The listing builds one solid part. Answer for the finished solid, in the listing's coordinates (mm). Coordinates: 2 decimals unless noted, no trailing zeros. Order: outer loops, then holes, each group sorted by start corner. A loop starts at its lowest first (then second) coordinate and runs counter-clockwise, first axis right, second up. Notation, with made-up numbers: (20, -9.75) - (58, -9.75) arc R6 cw to (58, 0.25) - close; hole circle Ø10 at (28.5, 12.5). An arc over 180 degrees is marked (long way). Use a Markdown table: item, result. Add a question column.
Item 1: The part is cut by section D-D, the plane y = 165.5. Give the vertices of the cut face in (x, z), then the cut area to 3 significant figures.
Item 2: Find the intervals of material crossed by line 1 along Z through (x, y) = (72, 80); line 2 along Y through (x, z) = (0, -162); line 3 along Y through (x, z) = (0, 104), in increasing order.
Item 3: The part is cut by section C-C, the plane y = 34. Give the vertices of the cut face in (x, z).
Item 4: Flat-ended cylindrical pins translate along their axes: P1, Ø17, axis at x = 197.99, y = 197.99, coming from the +Z side; P2, Ø15, axis at x = 77.78, y = -77.78, coming from the -Z side; P3, Ø21, axis at x = -77.78, y = 77.78, coming from the -Z side. Find the tip coordinate at first contact, or state that the pin passes through.
Item 5: The part is cut by section A-A, the plane x = 134. Give the vertices of the cut face in (y, z), then the cut area to 3 significant figures.
Item 6: The part is cut by section B-B, the plane z = 136. Give the vertices of the cut face in (x, y), then the cut area to 3 significant figures.
from build123d import *

# Parameters (mm, degrees)
SKETCH1_R               = 17.5
SKETCH1_R_2             = 6.5
BOSS_EXTRUDE1_DEPTH     = 280
SKETCH2_R               = 6.5
BOSS_EXTRUDE2_DEPTH     = 10
SKETCH3_R               = 6.5
BOSS_EXTRUDE3_DEPTH     = 10
MIRROR3_COPY_1_SKETCH_R = 6.5
MIRROR3_COPY_1_DEPTH    = 10
SKETCH4_R               = 6.5
BOSS_EXTRUDE4_DEPTH     = 5


with BuildPart() as part:
    # Sketch1 → Boss-Extrude1 (new, symmetric)
    with BuildSketch(Plane.XY):
        Circle(SKETCH1_R)
        Circle(SKETCH1_R_2, mode=Mode.SUBTRACT)
    extrude(amount=BOSS_EXTRUDE1_DEPTH, both=True)

    # Sketch2 → Boss-Extrude2 (add)
    with BuildSketch(Plane.XY.offset(210)):
        with BuildLine():
            Line((-12.374368671, 12.374368671), (192.686597873, 217.435335215))
            ThreePointArc((192.686597873, 217.435335215), (199.757665685, 220.364267403), (206.828733497, 217.435335215))
            Line((206.828733497, 217.435335215), (217.435335215, 206.828733497))
            ThreePointArc((217.435335215, 206.828733497), (220.364267403, 199.757665685), (217.435335215, 192.686597873))
            Line((217.435335215, 192.686597873), (12.374368671, -12.374368671))
            ThreePointArc((12.374368671, -12.374368671), (12.374368671, 12.374368671), (-12.374368671, 12.374368671))
        make_face()
        with Locations((197.989898732, 197.989898732)):
            Circle(SKETCH2_R, mode=Mode.SUBTRACT)
    boss_extrude2 = extrude(amount=-BOSS_EXTRUDE2_DEPTH)

    # Mirror1: Boss-Extrude2 across plane
    add(boss_extrude2.mirror(Plane.XY))

    # Sketch3 → Boss-Extrude3 (add)
    with BuildSketch(Plane.XY.offset(130)):
        with BuildLine():
            Line((12.374368671, 12.374368671), (-72.478445072, 97.227182413))
            ThreePointArc((-72.478445072, 97.227182413), (-79.549512883, 100.156114601), (-86.620580695, 97.227182413))
            Line((-86.620580695, 97.227182413), (-97.227182413, 86.620580695))
            ThreePointArc((-97.227182413, 86.620580695), (-100.156114601, 79.549512883), (-97.227182413, 72.478445072))
            Line((-97.227182413, 72.478445072), (-12.374368671, -12.374368671))
            ThreePointArc((-12.374368671, -12.374368671), (-12.374368671, 12.374368671), (12.374368671, 12.374368671))
        make_face()
        with Locations((-77.781745931, 77.781745931)):
            Circle(SKETCH3_R, mode=Mode.SUBTRACT)
    boss_extrude3 = extrude(amount=-BOSS_EXTRUDE3_DEPTH)

    # Mirror2: Boss-Extrude3 across plane
    add(boss_extrude3.mirror(Plane(origin=(0, 0, 102), x_dir=(1, 0, 0), z_dir=(0, 0, -1))))

    # Mirror3: Boss-Extrude3 across plane
    add(boss_extrude3.mirror(Plane.XY))

    # Mirror3 copy 1 sketch → Mirror3 copy 1 (add)
    with BuildSketch(Plane.XY.offset(-74)):
        with BuildLine():
            Line((12.374368671, 12.374368671), (-72.478445072, 97.227182413))
            ThreePointArc((-72.478445072, 97.227182413), (-79.549512883, 100.156114601), (-86.620580695, 97.227182413))
            Line((-86.620580695, 97.227182413), (-97.227182413, 86.620580695))
            ThreePointArc((-97.227182413, 86.620580695), (-100.156114601, 79.549512883), (-97.227182413, 72.478445072))
            Line((-97.227182413, 72.478445072), (-12.374368671, -12.374368671))
            ThreePointArc((-12.374368671, -12.374368671), (-12.374368671, 12.374368671), (12.374368671, 12.374368671))
        make_face()
        with Locations((-77.781745931, 77.781745931)):
            Circle(MIRROR3_COPY_1_SKETCH_R, mode=Mode.SUBTRACT)
    extrude(amount=-MIRROR3_COPY_1_DEPTH)

    # Sketch4 → Boss-Extrude4 (add, symmetric)
    with BuildSketch(Plane(origin=(0, 0, 102), x_dir=(-1, 0, 0), z_dir=(0, 0, -1))):
        with BuildLine():
            Line((-12.374368671, 12.374368671), (-97.227182413, -72.478445072))
            ThreePointArc((-97.227182413, -72.478445072), (-100.156114601, -79.549512883), (-97.227182413, -86.620580695))
            Line((-97.227182413, -86.620580695), (-86.620580695, -97.227182413))
            ThreePointArc((-86.620580695, -97.227182413), (-79.549512883, -100.156114601), (-72.478445072, -97.227182413))
            Line((-72.478445072, -97.227182413), (12.374368671, -12.374368671))
            ThreePointArc((12.374368671, -12.374368671), (-12.374368671, -12.374368671), (-12.374368671, 12.374368671))
        make_face()
        with Locations((-77.781745931, -77.781745931)):
            Circle(SKETCH4_R, mode=Mode.SUBTRACT)
    extrude(amount=BOSS_EXTRUDE4_DEPTH, both=True)


solid = part.part
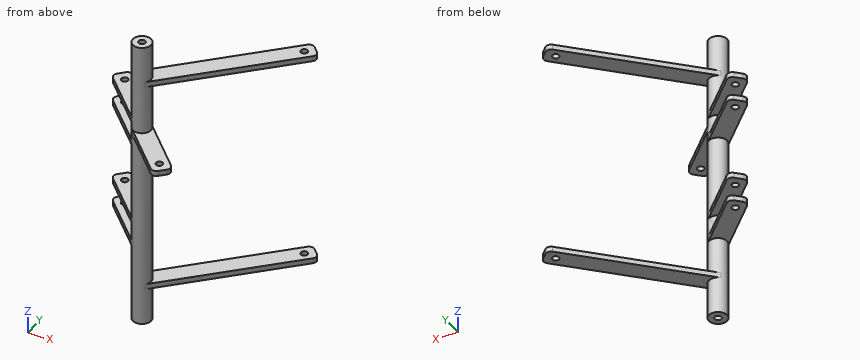
Solution:
| question | item | result |
|---|---|---|
| 1 | outline | (140.75, -210) - (190.25, -210) - (190.25, -200) - (140.75, -200) - close; (140.75, 200) - (190.25, 200) - (190.25, 210) - (140.75, 210) - close |
| 1 | area | 990 mm2 |
| 2 | line 1 | z = -210 to -200, 200 to 210 |
| 2 | line 2 | y = -17.5 to -6.5, 6.5 to 17.5 |
| 2 | line 3 | y = -24.75 to -6.5, 6.5 to 17.5 |
| 3 | outline | (-58.75, -130) - (-9.25, -130) - (-9.25, -120) - (-58.75, -120) - close; (-58.75, -84) - (-9.25, -84) - (-9.25, -74) - (-58.75, -74) - close; (-58.75, 74) - (-9.25, 74) - (-9.25, 84) - (-58.75, 84) - close; (-58.75, 120) - (-9.25, 120) - (-9.25, 130) - (-58.75, 130) - close; (9.25, -210) - (58.75, -210) - (58.75, -200) - (9.25, -200) - close; (9.25, 200) - (58.75, 200) - (58.75, 210) - (9.25, 210) - close |
| 4 | P1 | stops at z = 210 |
| 4 | P2 | stops at z = 97 |
| 4 | P3 | stops at z = -130 |
| 5 | outline | (109.25, -210) - (158.75, -210) - (158.75, -200) - (109.25, -200) - close; (109.25, 200) - (158.75, 200) - (158.75, 210) - (109.25, 210) - close |
| 5 | area | 990 mm2 |
| 6 | outline | circle Ø35 at (0, 0); hole circle Ø13 at (0, 0) |
| 6 | area | 829 mm2 |
